Here's how the part is built. I have some questions about the finished solid (model axes, mm). A direction names the side the tool comes from. Give positions to 0.01 mm unless a question says otherwise; leave off trailing zeros. Order: outer loops, then holes, each group sorted by start corner. A loop starts at its lowest first (then second) coordinate and runs counter-clockwise, first axis right, second up.
from build123d import *

# Parameters (mm, degrees)
SKETCH1_W           = 95.7
SKETCH1_H           = 95.7
BOSS_EXTRUDE1_DEPTH = 6.8
SKETCH2_W           = 206.7
SKETCH2_H           = 235.7
BOSS_EXTRUDE2_DEPTH = 6.8
SKETCH3_R           = 41
BOSS_EXTRUDE3_DEPTH = 3.3
SKETCH4_R           = 14.925
BOSS_EXTRUDE4_DEPTH = 6.25


with BuildPart() as part:
    # Sketch1 → Boss-Extrude1 (new body)
    with BuildSketch(Plane.XY):
        Rectangle(SKETCH1_W, SKETCH1_H)
    extrude(amount=BOSS_EXTRUDE1_DEPTH)

    # Sketch2 → Boss-Extrude2 (add)
    with BuildSketch(Plane.XY):
        with Locations((55.5, -10)):
            Rectangle(SKETCH2_W, SKETCH2_H)
    extrude(amount=-BOSS_EXTRUDE2_DEPTH)

    # Sketch3 → Boss-Extrude3 (add)
    with BuildSketch(Plane.XY.offset(6.8)):
        Circle(SKETCH3_R)
    extrude(amount=BOSS_EXTRUDE3_DEPTH)

    # Sketch4 → Boss-Extrude4 (add)
    with BuildSketch(Plane.XY.offset(10.1)):
        Circle(SKETCH4_R)
    extrude(amount=BOSS_EXTRUDE4_DEPTH)


solid = part.part
Q1. I need wall thicknesses on L1, parallel to Y at x = 34.5, z = 3.75; L2, parallel to Z at x = 52, y = -38; L3, parallel to Z at x = -34.5, y = 28. Which ranges of each line are inside material? Lowest first, please.
Filled sheet:
L1: y = -47.85 to 47.85
L2: z = -6.8 to 0
L3: z = -6.8 to 6.8
Q2. For faces 1 (the face through (-43, 1, 6.8)), 2 (the face through (-1, 47.85, 3)), 3 (the face through (-1, -47.85, 3)), which set-ups out of +Z, -Z, +X, -X, +Y, -Y let a thin tool reach every point of the face, with its end or its side?
Filled sheet:
face 1: +Z
face 2: +Z, +X, -X, +Y
face 3: +Z, +X, -X, -Y
Q3. I'm going to push flat-ended pins straight in: P1, Ø3.5, axis at y = 3, z = 3, coming from the +X side; P2, Ø3.5, axis at x = -19, z = 3.5, coming from the -Y side; P3, Ø1.5, axis at x = 5.5, z = 14, coming from the -Y side. Where does each tip first touch, or does it pass through?
Filled sheet:
P1: stops at x = 47.85
P2: stops at y = -47.85
P3: stops at y = -14.15
Q4. If we section it at B-B on y = 0: List the corners of the cut face in (x, z) for me (3 decimals).
Filled sheet:
outline: (-47.85, -6.8) - (158.85, -6.8) - (158.85, 0) - (47.85, 0) - (47.85, 6.8) - (41, 6.8) - (41, 10.1) - (14.925, 10.1) - (14.925, 16.35) - (-14.925, 16.35) - (-14.925, 10.1) - (-41, 10.1) - (-41, 6.8) - (-47.85, 6.8) - close
Q5. If we section it at C-C on y = 24.5: List the corners of the cut face in (x, z) for me, plus the area to 3 significant figures.
Filled sheet:
outline: (-47.85, -6.8) - (158.85, -6.8) - (158.85, 0) - (47.85, 0) - (47.85, 6.8) - (32.87, 6.8) - (32.87, 10.1) - (-32.87, 10.1) - (-32.87, 6.8) - (-47.85, 6.8) - close
area: 2,270 mm2
Q6. If we section it at A-A on x = 0: List the corners of the cut face in (y, z) for me (3 decimals).
Filled sheet:
outline: (-127.85, -6.8) - (107.85, -6.8) - (107.85, 0) - (47.85, 0) - (47.85, 6.8) - (41, 6.8) - (41, 10.1) - (14.925, 10.1) - (14.925, 16.35) - (-14.925, 16.35) - (-14.925, 10.1) - (-41, 10.1) - (-41, 6.8) - (-47.85, 6.8) - (-47.85, 0) - (-127.85, 0) - close
Q7. If we section it at D-D on x = 118.5: List the corners of the cut face in (y, z) for me, plus the area to 3 significant figures.
Filled sheet:
outline: (-127.85, -6.8) - (107.85, -6.8) - (107.85, 0) - (-127.85, 0) - close
area: 1,600 mm2
